Can you work these out from the model? Positions are in its coordinate system, mm. A direction names the side the tool comes from. Give positions to 0.01 mm unless a question says otherwise; leave off trailing zeros. Loops run counter-clockwise (first coordinate to the right, second up) from the corner with the lowest first, then second, coordinate; pieces in that order, holes last. Notation, with made-up numbers: M 6,47.25 L 16,47.25 A21 cw 16,55.25 Z; hole C -32,53.25 d4. An arc over 180 degrees is marked long. Put each result on its own line as item: value. Start each with the question number.
1) Please list where these lines run through material, in increasing order: line 1 along X through (y, z) = (1.75, -44); line 2 along X through (y, z) = (3.75, -56.5); line 3 along Z through (x, y) = (-203.5, 3). Write a range as from..to.
2) For faces 4 (the cylindrical face through (-136.89, -7.094, -7.219)), 5 (the cylindrical face through (-365.49, 7.094, -192.781)), 6 (the cylindrical face through (-284.34, 0.02, -15.35)), 7 (the cylindrical face through (-313.2, 0.02, -186.43)), 8 (the cylindrical face through (-292.906, 7.219, -100.98)), which set-ups out of +Z, -Z, +X, -X, +Y, -Y let a thin tool reach every point of the face, with its end or its side?
3) For P1, Ø1.5, axis at x = -348, y = -0.5, coming from the +Z side; P2, Ø0.9, axis at y = 0, z = -82, coming from the +X side; P3, Ø0.9, axis at x = -77, y = 0, coming from the -Z side, each with a flat end and sliding along its axis, tell me the tip position at first contact or that it passes through.
4) Imagine slicing it at B-B (z = -125). Write out the boundary of the cut face in (x, y).
5) If we mould it in two halves opening along Z, with no side actions, what happens to faces 1 (the cylindrical face through (-365.49, 7.219, -207.094)), 2 (the cylindrical face through (-307.094, -7.219, -100.98)), 3 (the cylindrical face through (-303.908, -0.021, -195.524))? For each: +Z half, -Z half, draft (parallel to the pull), parting line (faces both ways), or undercut.
6) Imagine slicing it at A-A (x = -248). Write out the boundary of the cut face in (y, z).
from build123d import *


with BuildPart() as part:
    # Sweep-Thin1: sweep along a path in Sketch1
    with BuildLine(Plane(origin=(0, 0, 0), x_dir=(1, 0, 0), z_dir=(0, 1, 0))) as sweep_thin1_path:
        Line((0, 0), (-270, 0))
        ThreePointArc((-270, 0), (-291.213203436, 8.786796564), (-300, 30))
        Line((-300, 30), (-300, 170))
        ThreePointArc((-300, 170), (-308.786796564, 191.213203436), (-330, 200))
        Line((-330, 200), (-400, 200))
    # Sketch2 → Sweep-Thin1 (sweep)
    with BuildSketch(Plane(origin=(0, 0, 0), x_dir=(0, 0, -1), z_dir=(1, 0, 0))):
        with BuildLine():
            Line((1.5, 9.5), (-1.5, 9.5))
            ThreePointArc((-1.5, 9.5), (-7.156854249, 7.156854249), (-9.5, 1.5))
            Line((-9.5, 1.5), (-9.5, -1.5))
            ThreePointArc((-9.5, -1.5), (-7.156854249, -7.156854249), (-1.5, -9.5))
            Line((-1.5, -9.5), (1.5, -9.5))
            ThreePointArc((1.5, -9.5), (7.156854249, -7.156854249), (9.5, -1.5))
            Line((9.5, -1.5), (9.5, 1.5))
            ThreePointArc((9.5, 1.5), (7.156854249, 7.156854249), (1.5, 9.5))
        make_face()
        with BuildLine():
            Line((1.5, 6.5), (-1.5, 6.5))
            ThreePointArc((-1.5, 6.5), (-5.035533906, 5.035533906), (-6.5, 1.5))
            Line((-6.5, 1.5), (-6.5, -1.5))
            ThreePointArc((-6.5, -1.5), (-5.035533906, -5.035533906), (-1.5, -6.5))
            Line((-1.5, -6.5), (1.5, -6.5))
            ThreePointArc((1.5, -6.5), (5.035533906, -5.035533906), (6.5, -1.5))
            Line((6.5, -1.5), (6.5, 1.5))
            ThreePointArc((6.5, 1.5), (5.035533906, 5.035533906), (1.5, 6.5))
        make_face(mode=Mode.SUBTRACT)
    sweep(path=sweep_thin1_path.line)


solid = part.part
Recorded:
1. line 1: -309.5..-306.49, -293.51..-290.5
1. line 2: -309.18..-305.97, -294.03..-290.82
1. line 3: -9.36..-6.27, 6.27..9.36
2. face 4: -Z, +X, -Y
2. face 5: +Z, -X, +Y
2. face 6: -Z, +X, +Y, -Y
2. face 7: none
2. face 8: -Z, +X, +Y
3. P1: z = -190.5
3. P2: x = -290.5
3. P3: z = -9.5
4. outline: M -309.5,-1.5 A8 ccw -301.5,-9.5 L -298.5,-9.5 A8 ccw -290.5,-1.5 L -290.5,1.5 A8 ccw -298.5,9.5 L -301.5,9.5 A8 ccw -309.5,1.5 Z; hole M -306.5,-1.5 A5 ccw -301.5,-6.5 L -298.5,-6.5 A5 ccw -293.5,-1.5 L -293.5,1.5 A5 ccw -298.5,6.5 L -301.5,6.5 A5 ccw -306.5,1.5 Z
5. face 1: -Z half
5. face 2: draft
5. face 3: undercut
6. outline: M -9.5,-1.5 A8 ccw -1.5,-9.5 L 1.5,-9.5 A8 ccw 9.5,-1.5 L 9.5,1.5 A8 ccw 1.5,9.5 L -1.5,9.5 A8 ccw -9.5,1.5 Z; hole M -6.5,-1.5 A5 ccw -1.5,-6.5 L 1.5,-6.5 A5 ccw 6.5,-1.5 L 6.5,1.5 A5 ccw 1.5,6.5 L -1.5,6.5 A5 ccw -6.5,1.5 Z
